Geometry: final body of the model. Coordinates: model frame, mm. A direction names the side the tool comes from. Give positions to 0.01 mm unless a question says otherwise; leave off trailing zeros. Order: outer loops, then holes, each group sorted by start corner. A loop starts at its lowest first (then second) coordinate and runs counter-clockwise, first axis right, second up. Notation, with made-up numbers: (73.5, 59.5) - (86.5, 59.5) arc R27 cw to (86.5, 82.5) - close; hole circle Ø2 at (74.5, -22.5). An arc over 180 degrees is marked (long way). Put each result on its own line as item: value. Start each with the question number.
1. Section B-B on y = -18. Return the cut outline in (x, z).
2. Mould query, pull axis X, two halves, no side actions, for faces 3 (the flat face through (-95, -1, -20)), 4 (the flat face through (-1.33, 34.79, -37.535)), 5 (the flat face through (-1, 0, -37.5)). Classes: pulls with the +X half, pulls with the -X half, needs draft (parallel to the pull), parting line crosses it, or undercut.
3. Set-up query: faces 1 (the flat face through (-1, -50, -17)), 2 (the flat face through (-1.295, 33.453, -35.223)). Return all of +Z, -Z, +X, -X, +Y, -Y with unobstructed straight access to the full face (end or side cutting, diameter ignored); none if empty.
4. First-contact query: P1, Ø10, axis at x = -29.5, y = 33, coming from the -Z side; P2, Ø5, axis at x = 63, y = 36.5, coming from the +Z side. Flat tips, straight axial feed; report the tip coordinate or a pass-through.
5. Ray query, line 1 along Y through (x, z) = (-63, -13); line 2 along X through (y, z) = (-15, -14); line 3 along Z through (x, y) = (73.5, 4). Return the intervals inside material, ascending. Write a range as from..to.
6. Section D-D on y = 25. Return the cut outline in (x, z), plus the area to 3 significant figures.
7. Section A-A on z = -5. Return the cut outline in (x, y).
8. Section C-C on x = 77.5. Return the cut outline in (y, z), plus the area to 3 significant figures.
from build123d import *

# Parameters (mm, degrees)
F0_W     = 190
F0_H     = 100
F1_DEPTH = 40
F2_SIZE2 = 30
F2_SIZE  = 5
F3_T     = -2.5


with BuildPart() as f1:
    # F0 (on Top) → F1 (new body)
    with BuildSketch(Plane.XY):
        Rectangle(F0_W, F0_H)
    extrude(amount=-F1_DEPTH)

    # F2
    f2_edges = [f1.edges().sort_by_distance(p)[0] for p in [
        (0, 50, -40),
        (0, -50, -40),
    ]]
    chamfer(f2_edges, length=F2_SIZE, length2=F2_SIZE2)

    # F3
    f3_openings = [f1.faces().sort_by_distance(p)[0] for p in [
        (0, 0, 0),
    ]]
    offset(amount=F3_T, openings=f3_openings)


solid = f1.part
Resolved:
1. outline: (-95, -40) - (95, -40) - (95, 0) - (92.5, 0) - (92.5, -37.5) - (-92.5, -37.5) - (-92.5, 0) - (-95, 0) - close
2. face 3: pulls with the -X half
2. face 4: needs draft
2. face 5: undercut
3. face 1: +Z, -Z, +X, -X, -Y
3. face 2: +Z
4. P1: z = -38.67
4. P2: z = -34.3
5. line 1: -50..-47.5, 47.5..50
5. line 2: -95..-92.5, 92.5..95
5. line 3: -40..-37.5
6. outline: (-95, -39.17) - (95, -39.17) - (95, 0) - (92.5, 0) - (92.5, -36.63) - (-92.5, -36.63) - (-92.5, 0) - (-95, 0) - close
6. area: 665 mm^2
7. outline: (-95, -50) - (95, -50) - (95, 50) - (-95, 50) - close; hole (-92.5, -47.5) - (92.5, -47.5) - (92.5, 47.5) - (-92.5, 47.5) - close
8. outline: (-50, -35) - (-20, -40) - (20, -40) - (50, -35) - (50, 0) - (47.5, 0) - (47.5, -32.88) - (19.79, -37.5) - (-19.79, -37.5) - (-47.5, -32.88) - (-47.5, 0) - (-50, 0) - close
8. area: 415 mm^2
